Design review of the part built by this model. Coordinates are the model's own, in mm. A direction names the side the tool comes from. Give positions to 0.01 mm unless a question says otherwise; leave off trailing zeros. Order: outer loops, then holes, each group sorted by start corner. A loop starts at its lowest first (then second) coordinate and runs counter-clockwise, first axis right, second up. Notation, with made-up numbers: (66.25, 28.5) -> (121.25, 28.5) arc R14 cw to (121.25, 45.5) -> close; hole circle Ø6 at (-34, 21). An arc over 180 degrees is marked (long way). Return JSON: item names as keys, results as strings.
```python
from build123d import *

# Parameters (mm, degrees)
SKETCH1_W               = 75
SKETCH1_H               = 50
SKETCH1_R               = 5.1
SKETCH1_R_2             = 7.6
BOSS_EXTRUDE1_DEPTH     = 5
SKETCH2_W               = 12.5
SKETCH2_H               = 40
BOSS_EXTRUDE2_DEPTH     = 12.5
SKETCH3_R               = 4
CUT_EXTRUDE1_DEPTH      = 92.821838361
SKETCH4_W               = 50
SKETCH4_H               = 30
BOSS_EXTRUDE3_DEPTH     = 5
SKETCH5_R               = 2
SKETCH5_R_2             = 11
CUT_EXTRUDE2_DEPTH      = 92.001373616
SKETCH6_W               = 32
SKETCH6_H               = 12
BOSS_EXTRUDE4_DEPTH     = 2
BOSS_EXTRUDE6_DEPTH     = 32
SKETCH9_W               = 6
SKETCH9_H               = 25.9
BOSS_EXTRUDE7_DEPTH     = 2
BOSS_EXTRUDE8_DEPTH     = 6
CUT_EXTRUDE3_DEPTH      = 97.571217244
CUT_EXTRUDE3_DEPTH_BACK = 97.571217244
SKETCH11_R              = 2
SKETCH11_R_2            = 1.5
SKETCH13_R              = 3.7
SKETCH13_R_2            = 2.75
SKETCH13_W              = 5.5
SKETCH13_H              = 1.674207078
CUT_EXTRUDE4_DEPTH      = 94.813645063


with BuildPart() as part:
    # Sketch1 → Boss-Extrude1 (new body)
    with BuildSketch(Plane(origin=(0, 0, 0), x_dir=(1, 0, 0), z_dir=(0, 1, 0))):
        with Locations((37.5, 25)):
            Rectangle(SKETCH1_W, SKETCH1_H)
        with Locations(Location((24.5, 32.5, 0), (0, 0, 270))):
            Circle(SKETCH1_R, mode=Mode.SUBTRACT)
        with Locations(Location((50.5, 32.5, 0), (0, 0, 270))):
            Circle(SKETCH1_R_2, mode=Mode.SUBTRACT)
    extrude(amount=BOSS_EXTRUDE1_DEPTH)

    # Sketch2 → Boss-Extrude2 (add)
    with BuildSketch(Plane(origin=(0, 5, 0), x_dir=(1, 0, 0), z_dir=(0, 1, 0))):
        with Locations((6.25, 30)):
            Rectangle(SKETCH2_W, SKETCH2_H)
        with Locations((68.75, 30)):
            Rectangle(SKETCH2_W, SKETCH2_H)
    extrude(amount=BOSS_EXTRUDE2_DEPTH)

    # Sketch3 → Cut-Extrude1 (cut, through all)
    with BuildSketch(Plane(origin=(0, 0, -50), x_dir=(-1, 0, 0), z_dir=(0, 0, -1))):
        with Locations((-68.75, 11.25)):
            Circle(SKETCH3_R)
        with Locations((-6.25, 11.25)):
            Circle(SKETCH3_R)
        Polygon((-72.525126266, 17.5), (-75, 17.5), (-75, 15.025126266), align=None)
        Polygon((-62.5, 17.5), (-64.974873734, 17.5), (-62.5, 15.025126266), align=None)
        Polygon((-12.5, 15.025126266), (-12.5, 17.5), (-10.025126266, 17.5), align=None)
        Polygon((0, 15.025126266), (-2.474873734, 17.5), (0, 17.5), align=None)
    extrude(amount=-CUT_EXTRUDE1_DEPTH, mode=Mode.SUBTRACT)

    # Sketch4 → Boss-Extrude3 (add)
    with BuildSketch(Plane(origin=(0, 5, 0), x_dir=(1, 0, 0), z_dir=(0, 1, 0))):
        with Locations((37.5, -15)):
            Rectangle(SKETCH4_W, SKETCH4_H)
    extrude(amount=-BOSS_EXTRUDE3_DEPTH)

    # Sketch5 → Cut-Extrude2 (cut, through all)
    with BuildSketch(Plane(origin=(0, 5, 0), x_dir=(1, 0, 0), z_dir=(0, 1, 0))):
        with Locations(Location((22, -24.5, 0), (0, 0, 270))):
            Circle(SKETCH5_R)
        with Locations(Location((22, 6.5, 0), (0, 0, 90))):
            Circle(SKETCH5_R)
        with Locations(Location((53, 6.5, 0), (0, 0, 270))):
            Circle(SKETCH5_R)
        with Locations(Location((53, -24.5, 0), (0, 0, 90))):
            Circle(SKETCH5_R)
        with Locations(Location((37.5, -9, 0), (0, 0, 270))):
            Circle(SKETCH5_R_2)
    extrude(amount=-CUT_EXTRUDE2_DEPTH, mode=Mode.SUBTRACT)

    # Sketch6 → Boss-Extrude4 (add)
    with BuildSketch(Plane(origin=(0, 5, 0), x_dir=(1, 0, 0), z_dir=(0, 1, 0))):
        with Locations((37.5, 18.1)):
            Rectangle(SKETCH6_W, SKETCH6_H)
    extrude(amount=BOSS_EXTRUDE4_DEPTH)

    # Sketch8 → Boss-Extrude6 (add)
    with BuildSketch(Plane(origin=(53.5, 0, 0), x_dir=(0, 0, -1), z_dir=(1, 0, 0))):
        Polygon((24.1, 7), (12.1, 7), (12.1, 31), align=None)
    extrude(amount=-BOSS_EXTRUDE6_DEPTH)

    # Sketch9 → Boss-Extrude7 (add)
    with BuildSketch(Plane(origin=(0, 5, 0), x_dir=(1, 0, 0), z_dir=(0, 1, 0))):
        with Locations((37.5, 37.05)):
            Rectangle(SKETCH9_W, SKETCH9_H)
    extrude(amount=BOSS_EXTRUDE7_DEPTH)

    # Sketch10 → Boss-Extrude8 (add)
    with BuildSketch(Plane.ZY.offset(-34.5)):
        Polygon((-50, 7), (-12.1, 31), (-24.1, 7), align=None)
    extrude(amount=-BOSS_EXTRUDE8_DEPTH)

    # Sketch11 → Cut-Extrude3 (cut, two sides: drawn at the far end of the back side and taken through both)
    with BuildSketch(Plane(origin=(0, 5, 5), x_dir=(1, 0, 0), z_dir=(0, 1, 0)).offset(-CUT_EXTRUDE3_DEPTH_BACK)):
        with Locations(Location((50.5, 25.43, 0), (0, 0, 270))):
            Circle(SKETCH11_R)
        with Locations(Location((50.5, 49.565, 0), (0, 0, 270))):
            Circle(SKETCH11_R)
        with Locations(Location((24.5, 45.5, 0), (0, 0, 270))):
            Circle(SKETCH11_R_2)
        with Locations(Location((16.5, 37.5, 0), (0, 0, 270))):
            Circle(SKETCH11_R_2)
        with Locations(Location((32.5, 37.5, 0), (0, 0, 90))):
            Circle(SKETCH11_R_2)
        with Locations(Location((24.5, 29.5, 0), (0, 0, 195.466009953))):
            Circle(SKETCH11_R_2)
    extrude(amount=CUT_EXTRUDE3_DEPTH + CUT_EXTRUDE3_DEPTH_BACK, mode=Mode.SUBTRACT)

    # Sketch13 → Cut-Extrude4 (cut, through all)
    with BuildSketch(Plane(origin=(0, 5, 0), x_dir=(1, 0, 0), z_dir=(0, 1, 0))):
        with Locations((50.5, 20.43)):
            Circle(SKETCH13_R)
        with Locations((24.5, 24.5)):
            Circle(SKETCH13_R_2)
        with Locations((50.75, 23.262896461)):
            Rectangle(SKETCH13_W, SKETCH13_H)
    extrude(amount=CUT_EXTRUDE4_DEPTH, mode=Mode.SUBTRACT)


solid = part.part
```
Item 1: Mouldability with a two-part tool opening along Z and no side actions: class faces 4 (the face through (11.245, 16.28, -30.28)), 5 (the face through (28.1, 19.2, -18)), 6 (the face through (46.775, 2.535, 14.914)) as released by +Z, released by -Z, zero draft, split by the parting line, or undercut.
Result set:
{"face 4": "zero draft", "face 5": "released by -Z", "face 6": "undercut"}
Item 2: For pin 1 (5 mm diameter, centred on y = 25.5, z = -14.5, fed in from -X); pin 2 (5.5 mm diameter, centred on y = 2, z = 13.5, fed in from -X); pin 3 (12 mm diameter, centred on x = 27.5, z = -9.5, fed in from +Y), all flat-tipped, find the tip position at first contact; note any pin that passes through.
Result set:
{"pin 1": "stops at x = 21.5", "pin 2": "stops at x = 12.5", "pin 3": "stops at y = 31"}
Item 3: Wall thickness on L1, parallel to X at y = 3.1, z = 24.5; L2, parallel to X at y = 9.5, z = -36; L3, parallel to X at y = 2.5, z = -8: over which ranges is each line inside the solid? List them lowest first. Write a range as [from, to].
Result set:
{"L1": "x = [12.5, 20], [24, 51], [55, 62.5]", "L2": "x = [0, 2.65], [9.85, 12.5], [34.5, 40.5], [62.5, 65.15], [72.35, 75]", "L3": "x = [0, 20.68], [23.32, 51.68], [54.32, 75]"}
Item 4: Add section B-B (z = -32.5). Give the number of separate pieces and of enclosed holes in the cut face, plus the area to 3 significant figures.
Result set:
{"separate pieces": "5", "enclosed holes": "2", "area": "496 mm^2"}
Item 5: Add section D-D (y = 14). Give the boundary of the cut face in (x, z).
Result set:
{"outline": "(0, -50) -> (3.35, -50) -> (3.35, -10) -> (0, -10) -> close; (9.15, -50) -> (12.5, -50) -> (12.5, -10) -> (9.15, -10) -> close; (21.5, -20.6) -> (34.5, -20.6) -> (34.5, -38.95) -> (40.5, -38.95) -> (40.5, -20.6) -> (46.8, -20.6) arc R3.7 cw to (53.5, -18.26) -> (53.5, -12.1) -> (21.5, -12.1) -> close; (62.5, -50) -> (65.85, -50) -> (65.85, -10) -> (62.5, -10) -> close; (71.65, -50) -> (75, -50) -> (75, -10) -> (71.65, -10) -> close"}
Item 6: Machinability: for faces 1 (the face through (69, 2, 0)), 2 (the face through (6, 2, 0)), 3 (the face through (34.5, 15, -31)), which of the approach directions +Z, -Z, +X, -X, +Y, -Y give a long, thin tool a straight path to every point of the face, cutting with its end or side? Answer none if there is none.
Result set:
{"face 1": "+Z, +X, +Y, -Y", "face 2": "+Z, -X, +Y, -Y", "face 3": "-Z, +Y"}
Item 7: Add section A-A (x = 6.25). Give the boundary of the cut face in (y, z).
Result set:
{"outline": "(0, -50) -> (7.25, -50) -> (7.25, -10) -> (5, -10) -> (5, 0) -> (0, 0) -> close; (15.25, -50) -> (17.5, -50) -> (17.5, -10) -> (15.25, -10) -> close"}
